Design review of the part built by this model. Coordinates are the model's own, in mm. A direction names the side the tool comes from. Coordinates: 2 decimals unless noted, no trailing zeros. Write each loop counter-clockwise with the first axis right and the second up, starting at its lowest first coordinate (ties: lowest second). Pieces come first, ordered by that corner, then holes. Notation, with made-up numbers: (1.25, 5.25) - (52.25, 5.25) arc R21 cw to (52.25, 29.25) - close; hole circle Ø9 at (68.25, -20.5). An arc over 180 degrees is marked (long way). One line per item, written item: value.
from build123d import *

# Parameters (mm, degrees)
EXTRUDE_1_DEPTH     = 5
SKETCH_3_W          = 5
SKETCH_3_H          = 6
EXTRUDE_2_DEPTH     = 5
SKETCH_2_R          = 1.55
CUT_EXTRUDE_1_DEPTH = 43.720018727
CHAMFER_1_SIZE      = 0.5


with BuildPart() as part:
    # ｽｹｯﾁ1 → ﾎﾞｽ - 押し出し1 (new body)
    with BuildSketch(Plane.XY):
        with BuildLine():
            Line((0, 30), (18, 30))
            Line((18, 30), (18, 24))
            Line((18, 24), (12, 24))
            Line((12, 24), (12, 27))
            Line((12, 27), (0, 27))
            ThreePointArc((0, 27), (-27, 0), (0, -27))
            Line((0, -27), (12, -27))
            Line((12, -27), (12, -24))
            Line((12, -24), (18, -24))
            Line((18, -24), (18, -30))
            Line((18, -30), (0, -30))
            ThreePointArc((0, -30), (-30, 0), (0, 30))
        make_face()
    extrude(amount=EXTRUDE_1_DEPTH)

    # ｽｹｯﾁ3 → ﾎﾞｽ - 押し出し2 (add)
    with BuildSketch(Plane.XY.offset(5)):
        with Locations((20.5, -27)):
            Rectangle(SKETCH_3_W, SKETCH_3_H)
        with Locations((20.5, 27)):
            Rectangle(SKETCH_3_W, SKETCH_3_H)
    extrude(amount=-EXTRUDE_2_DEPTH)

    # ｽｹｯﾁ2 → ｶｯﾄ - 押し出し1 (cut, through all)
    with BuildSketch(Plane.XY.offset(5)):
        with Locations((20, -27)):
            Circle(SKETCH_2_R)
        with Locations((20, 27)):
            Circle(SKETCH_2_R)
    extrude(amount=-CUT_EXTRUDE_1_DEPTH, mode=Mode.SUBTRACT)

    # 面取り1
    chamfer_1_edges = [part.edges().sort_by_distance(p)[0] for p in [
        (11.5, 30, 0),
        (17.5, 24, 0),
        (12, 25.5, 0),
        (6, 27, 0),
        (-27, 0, 0),
        (17.5, -24, 5),
        (6, -27, 0),
        (12, -25.5, 0),
        (17.5, -24, 0),
        (11.5, -30, 0),
        (-30, 0, 0),
        (12, -25.5, 5),
        (6, -27, 5),
        (-27, 0, 5),
        (6, 27, 5),
        (12, 25.5, 5),
        (17.5, 24, 5),
        (23, -27, 5),
        (23, -27, 0),
        (11.5, 30, 5),
        (-30, 0, 5),
        (23, 27, 5),
        (23, 27, 0),
        (18.45, -27, 0),
        (18.45, -27, 5),
        (18.45, 27, 0),
        (18.45, 27, 5),
        (11.5, -30, 5),
    ]]
    chamfer(chamfer_1_edges, length=CHAMFER_1_SIZE)


solid = part.part
1. Consider section A-A, the plane x = 14.5. Write out the cut boundary in (y, z), then the cut area to 3 significant figures.
Answer block:
outline: (-30, 0.5) - (-29.5, 0) - (-24.5, 0) - (-24, 0.5) - (-24, 4.5) - (-24.5, 5) - (-29.5, 5) - (-30, 4.5) - close; (24, 0.5) - (24.5, 0) - (29.5, 0) - (30, 0.5) - (30, 4.5) - (29.5, 5) - (24.5, 5) - (24, 4.5) - close
area: 59.0 mm^2
2. Consider section C-C, the plane x = 20. Give the number of separate pieces and of enclosed holes in the cut face, then the cut area to 3 significant figures.
Answer block:
separate pieces: 4
enclosed holes: 0
area: 27.0 mm^2
3. Consider section D-D, the plane y = 0. Write out the cut boundary in (x, z).
Answer block:
outline: (-30, 0.5) - (-29.5, 0) - (-27.5, 0) - (-27, 0.5) - (-27, 4.5) - (-27.5, 5) - (-29.5, 5) - (-30, 4.5) - close
4. For faces 1 (the face through (12, -26, 2)), 2 (the face through (-27.129, 0.597, 0.365)), 3 (the face through (18, 24, 2)), 4 (the face through (11, -30, 3)), list the 3-axis set-ups (+Z, -Z, +X, -X, +Y, -Y) from which the entire face can be reached by the end or side of a thin tool; tool diameter is ignored.
Answer block:
face 1: +Z, -Z
face 2: -Z
face 3: +Z, -Z, +X
face 4: +Z, -Z, +X, -X, -Y
5. Consider section B-B, the plane z = 2.75. Write out the cut boundary in (x, y).
Answer block:
outline: (0, -30) - (23, -30) - (23, -24) - (12, -24) - (12, -27) - (0, -27) arc R27 cw to (0, 27) - (12, 27) - (12, 24) - (23, 24) - (23, 30) - (0, 30) arc R30 ccw to start; hole circle Ø3.1 at (20, -27); hole circle Ø3.1 at (20, 27)
6. Wall thickness on line 1 along Y through (x, z) = (20, 3.65); line 2 along Y through (x, z) = (17.5, 2.65); line 3 along Y through (x, z) = (9, 3.65): over which ranges is each line inside the solid? List them lowest first.
Answer block:
line 1: y = -30 to -28.55, -25.45 to -24, 24 to 25.45, 28.55 to 30
line 2: y = -30 to -24, 24 to 30
line 3: y = -30 to -27, 27 to 30
7. Mouldability with a two-part tool opening along X and no side actions: class faces 5 (the face through (-29.635, 0.652, 4.858)), 6 (the face through (-27, 7, 5)), 7 (the face through (-26.993, 0.594, 2.472)), 8 (the face through (12, 25, 2)) as released by +X, released by -X, zero draft, split by the parting line, or undercut.
Answer block:
face 5: released by -X
face 6: zero draft
face 7: undercut
face 8: undercut
8. Insertion check: pin 1 Ø1.5 at (y, z) = (25, 3) entering from -X; pin 2 Ø2.5 at (y, z) = (-26, 3.5) entering from -X; pin 3 Ø4 at (x, y) = (20, -27) entering from -Z. Each pin has a flat end and moves straight along its axis. Give the tip position at first contact, or say it passes through.
Answer block:
pin 1: stops at x = -17.66
pin 2: stops at x = -16.95
pin 3: stops at z = 0.05
